Geometry: see drawing. Coordinates: mm, zero at the bounding-box minimum. Round coordinates to 2 decimals unless told otherwise and drop trailing zeros. Loops run counter-clockwise (first coordinate to the right, second up) from the corner with the lowest first, then second, coordinate; pieces in that order, holes last.
(1) Section A-A, the plane x = 7. Return the cut outline in (y, z), plus the area to 3 significant figures.
(2) Section B-B, the plane y = 4.2. Return the cut outline in (x, z).
(3) Section C-C, the plane x = 10. Return the cut outline in (y, z).
(4) Mould query, pull axis X, two halves, no side actions, for the marked faces 1, 2 and 3. Classes: pulls with the +X half, pulls with the -X half, needs draft (parallel to the pull), parting line crosses it, or undercut.
(5) Material intervals for probe 1 along X at (y, z) = (2.3, 7); probe 2 along Z at (x, y) = (7, 2); probe 3 along Z at (x, y) = (8.25, 0.85), sorted ascending.
(6) Section D-D, the plane z = 3. Return the cut outline in (x, y), plus the area to 3 significant figures.
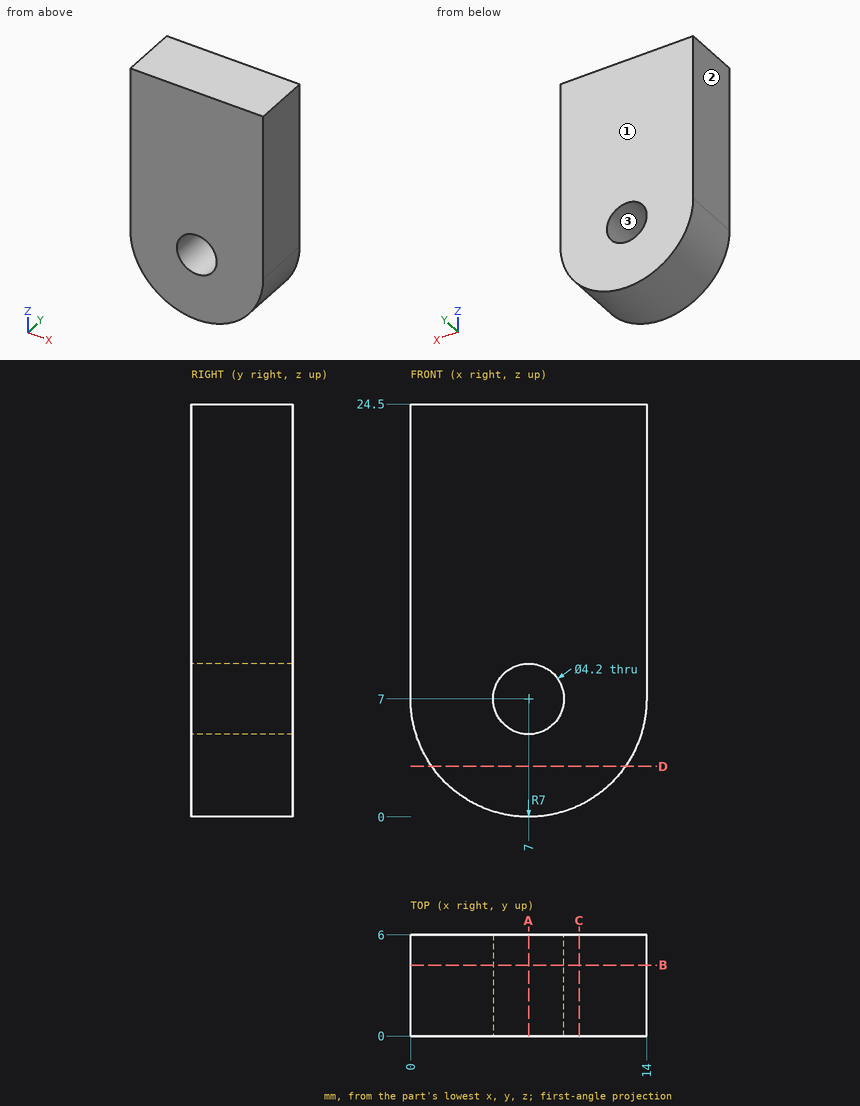
Output values:
1. outline: (0, 0) - (6, 0) - (6, 4.9) - (0, 4.9) - close; (0, 9.1) - (6, 9.1) - (6, 24.5) - (0, 24.5) - close
1. area: 122 mm2
2. outline: (0, 7) arc R7 ccw to (14, 7) - (14, 24.5) - (0, 24.5) - close; hole circle Ø4.2 at (7, 7)
3. outline: (0, 0.68) - (6, 0.68) - (6, 24.5) - (0, 24.5) - close
4. face 1: needs draft
4. face 2: pulls with the -X half
4. face 3: undercut
5. probe 1: x = 0 to 4.9, 9.1 to 14
5. probe 2: z = 0 to 4.9, 9.1 to 24.5
5. probe 3: z = 0.11 to 5.31, 8.69 to 24.5
6. outline: (1.26, 0) - (12.74, 0) - (12.74, 6) - (1.26, 6) - close
6. area: 68.9 mm2
